```python
from build123d import *

# Parameters (mm, degrees)
SKETCH1_W               = 635
SKETCH1_H               = 101.6
BOSS_EXTRUDE1_DEPTH     = 9.525
CUT_EXTRUDE1_DEPTH      = 644.147172601
CUT_EXTRUDE1_DEPTH_BACK = 9.525
CUT_EXTRUDE1_START      = 60.325
SKETCH2_W               = 1.5875
SKETCH2_H               = 50.8
CUT_EXTRUDE4_DEPTH      = 644.147172601
CUT_EXTRUDE4_DEPTH_BACK = 644.147172601
SKETCH3_R               = 6.35
SKETCH5_W               = 50.8
SKETCH5_H               = 101.6
CUT_EXTRUDE5_DEPTH      = 1.5875


with BuildPart() as part:
    # Sketch1 → Boss-Extrude1 (new body)
    with BuildSketch(Plane.XY):
        with Locations((317.5, 50.8)):
            Rectangle(SKETCH1_W, SKETCH1_H)
    extrude(amount=BOSS_EXTRUDE1_DEPTH)

    # Sketch2 → Cut-Extrude1 (cut, two sides: drawn at the far end of the back side and taken through both)
    with BuildSketch(Plane(origin=(0, 0, 0), x_dir=(0, 0, -1), z_dir=(1, 0, 0)).offset(CUT_EXTRUDE1_START - CUT_EXTRUDE1_DEPTH_BACK)):
        with Locations((-0.79375, 50.8)):
            Rectangle(SKETCH2_W, SKETCH2_H)
    extrude(amount=CUT_EXTRUDE1_DEPTH + CUT_EXTRUDE1_DEPTH_BACK, mode=Mode.SUBTRACT)

    # Sketch3 → Cut-Extrude4 (cut, two sides: drawn at the far end of the back side and taken through both)
    with BuildSketch(Plane(origin=(0, 0, 0), x_dir=(-1, 0, 0), z_dir=(0, 0, -1)).offset(-CUT_EXTRUDE4_DEPTH_BACK)):
        with Locations((-25.4, 88.9)):
            Circle(SKETCH3_R)
        with Locations((-114.3, 88.9)):
            Circle(SKETCH3_R)
        with Locations((-114.3, 12.7)):
            Circle(SKETCH3_R)
        with Locations((-25.4, 12.7)):
            Circle(SKETCH3_R)
    extrude(amount=CUT_EXTRUDE4_DEPTH + CUT_EXTRUDE4_DEPTH_BACK, mode=Mode.SUBTRACT)

    # Sketch5 → Cut-Extrude5 (cut)
    with BuildSketch(Plane(origin=(0, 0, 0), x_dir=(-1, 0, 0), z_dir=(0, 0, -1))):
        with Locations((-76.2, 50.8)):
            Rectangle(SKETCH5_W, SKETCH5_H)
    extrude(amount=-CUT_EXTRUDE5_DEPTH, mode=Mode.SUBTRACT)


solid = part.part
```
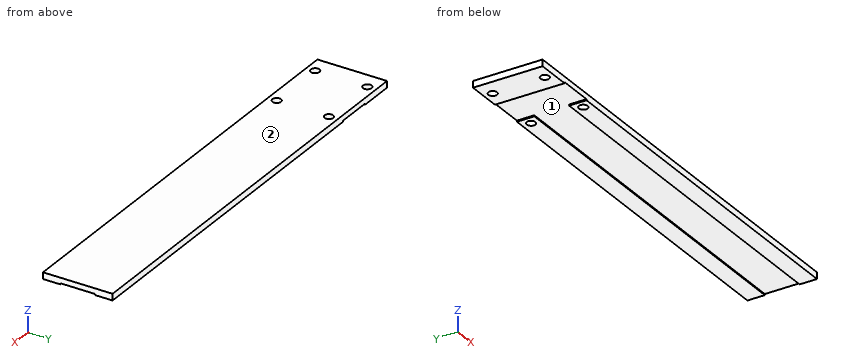
Geometry check sheet. Reference: the model listing, model coordinates, mm. Face numbers are marked on the shaded views. Give positions to 0.01 mm unless a question says otherwise; leave off trailing zeros. Write each loop counter-clockwise with the first axis right and the second up, starting at its lowest first coordinate (ties: lowest second). Pieces come first, ordered by that corner, then holes.
1) Release check for a two-part mould opening along Y. For the marked faces 1 and 2 record: pulls with the +Y half, pulls with the -Y half, needs draft (parallel to the pull), parting line crosses it, or undercut.
2) Material ranges on L1, parallel to X at y = 12.7, z = 4.25; L2, parallel to Y at x = 114.3, z = 3.5; L3, parallel to Y at x = 202.5, z = 1, recorded low to high.
3) Gauge pin test, flat ends, axial feed: pin 1 (0.5 mm diameter, centred on y = 30, z = 1, fed in from +X); pin 2 (1.5 mm diameter, centred on x = 170, y = 30, fed in from -Z). Record the tip position at first contact, or that the pin passes through.
4) Section check C-C, the plane x = 188. Record the boundary of the cut face in (y, z) (1 decimal), and give its area (3 significant figures).
5) Section check B-B, the plane y = 12.7. State how many separate pieces and enclosed holes the cut face has, and give its area (3 significant figures).
6) Section check A-A, the plane x = 25.4. Record the boundary of the cut face in (y, z) (3 decimals), and give its area (3 significant figures).
Computed:
1. face 1: undercut
1. face 2: needs draft
2. L1: x = 0 to 19.05, 31.75 to 107.95, 120.65 to 635
2. L2: y = 0 to 6.35, 19.05 to 82.55, 95.25 to 101.6
2. L3: y = 0 to 25.4, 76.2 to 101.6
3. pin 1: stops at x = 50.8
3. pin 2: stops at z = 1.59
4. outline: (0, 0) - (25.4, 0) - (25.4, 1.6) - (76.2, 1.6) - (76.2, 0) - (101.6, 0) - (101.6, 9.5) - (0, 9.5) - close
4. area: 887 mm2
5. separate pieces: 3
5. enclosed holes: 0
5. area: 5,730 mm2
6. outline: (0, 0) - (6.35, 0) - (6.35, 9.525) - (0, 9.525) - close; (19.05, 0) - (82.55, 0) - (82.55, 9.525) - (19.05, 9.525) - close; (95.25, 0) - (101.6, 0) - (101.6, 9.525) - (95.25, 9.525) - close
6. area: 726 mm2
